Autodesk Inventor part; units mm, degrees
ref_plane "YZ Plane" through (0, 0, 0) normal (1, 0, 0) x (0, 1, 0)
ref_plane "XZ Plane" through (0, 0, 0) normal (0, 1, 0) x (-1, 0, 0)
ref_plane "XY Plane" through (0, 0, 0) normal (0, 0, 1) x (1, 0, 0)
sketch "スケッチ1" plane through (0, 0, 0) normal (0, 1, 0) x (-1, 0, 0)
  circle A0 centre (56.6667, -3.3333) radius 2
  circle A1 centre (6.6667, -1.3333) radius 2
  arc A2 (27.618, -9.313) -> (80.2911, 0.2239) centre (24.5838, 157.671) ccw
  arc A3 (20.5062, -9.2317) -> (27.618, -9.313) centre (25.435, 110.8283) ccw
  arc A4 (7.5483, -6.9284) -> (20.5062, -9.2317) centre (22.5133, 39.66) ccw
  arc A5 (0.14, -3.2897) -> (7.5483, -6.9284) centre (16.2383, 20.125) ccw
  arc A6 (-1.8521, -1.3552) -> (0.14, -3.2897) centre (4.8333, 3.5367) ccw
  arc A7 (-0.4054, 2.2589) -> (-1.8521, -1.3552) centre (0, 0) ccw
  arc A8 (5.081, 2.7563) -> (-0.4054, 2.2589) centre (5.1833, -28.88) ccw
  arc A9 (23.6457, 1.9287) -> (5.081, 2.7563) centre (5.71, -191.7767) ccw
  arc A10 (23.6457, 1.9287) -> (35.0642, 0.89) centre (351.2983, 3540.5833) ccw
  arc A11 (35.0642, 0.89) -> (56.4197, -0.0064) centre (55.24, 226.7233) ccw
  arc A12 (56.4197, -0.0064) -> (79.9865, 1.514) centre (55.3817, 199.4967) ccw
  arc A13 (80.2911, 0.2239) -> (79.9865, 1.514) centre (80.0687, 0.8524) ccw
extrude "押し出し1" add sketch "スケッチ1" along normal mid plane 250 contours A0 | A1 | A3 A4 A5 A6 A7 A8 A9 A10 A11 A12 A13 A2
ref_plane "作業平面1" through (-121.5758, 135, -17.9326) normal (0.516, 0, -0.8566) x (0.8566, 0, 0.516)
sketch "スケッチ4" plane through (-121.5758, 135, -17.9326) normal (0.516, 0, -0.8566) x (0.8566, 0, 0.516)
  arc A0 (90, 35) -> (0, 0) centre (90, -98.2143) ccw
  line L0 (183.3333, 35) -> (90, 35)
  line L1 (183.3333, 35) -> (183.3333, 0)
  line L2 (183.3333, 0) -> (0, 0)
  point P0 (113.3913, 135)
extrude "押し出し4" cut sketch "スケッチ4" along normal through all
properties part number "newsubflap_top"
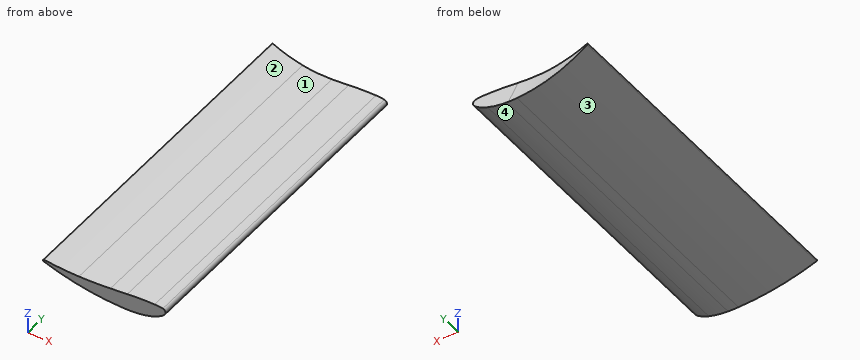
The model under review builds one solid part; all positions refer to its coordinate system, in mm. Face numbers are marked on the shaded views. Give positions to 0.01 mm unless a question says otherwise; leave off trailing zeros. Write each loop counter-clockwise with the first axis right and the second up, starting at its lowest first coordinate (ties: lowest second). Pieces come first, ordered by that corner, then holes. Notation, with made-up numbers: M 20.5,-25 L 33.5,-25 A20 ccw 33.5,4 Z; hole C 85,9 d1. An arc over 180 degrees is marked long. One line per question, with ' | ' between items. Start each with the question number.
Item 1: For pin 1 (3 mm diameter, centred on x = -9, z = -3, fed in from +Y); pin 2 (12 mm diameter, centred on x = -14, y = 65, fed in from +Z); pin 3 (1.5 mm diameter, centred on x = -40.5, z = -2.5, fed in from +Y), all flat-tipped, find the tip position at first contact; note any pin that passes through.
Item 2: Wall thickness on line 1 (Y direction, x = -3, z = -1.5); line 2 (Y direction, x = -34, z = -1.25); line 3 (Z direction, x = -74.5, y = -21): over which ranges is each line inside the solid? List them lowest first. Write a range as from..to.
Item 3: Draft analysis for pull direction X (two halves, no side actions). For the marked faces 1, 2, 3 and 4, state which applies: released by +X, released by -X, zero draft, split by the parting line, or undercut.
Item 4: We need section B-B on x = -18.5. Write out the cut boundary in (y, z).
Item 5: We need section A-A on y = -67. Write out the cut boundary in (x, z).
Results found:
1) pin 1: stops at y = 100 | pin 2: stops at z = 2.74 | pin 3: stops at y = 100.67
2) line 1: y = -125..100 | line 2: y = -125..100.15 | line 3: z = -1.71..0.91
3) face 1: undercut | face 2: undercut | face 3: released by -X | face 4: released by +X
4) outline: M -125,-9.11 L 100,-9.11 L 100,2.34 L -125,2.34 Z
5) outline: M -80.29,0.22 A167.02 ccw -27.62,-9.31 A120.16 ccw -20.51,-9.23 A48.93 ccw -7.55,-6.93 A28.41 ccw -0.14,-3.29 A8.29 ccw 1.85,-1.36 A2.29 ccw 0.41,2.26 A31.63 ccw -5.08,2.76 A194.55 ccw -23.65,1.93 A3557.02 cw -35.06,0.89 A226.74 cw -56.42,-0.01 A199.49 cw -79.99,1.51 A0.67 ccw Z
